Build history of the part. All positions in model axes, mm. A direction names the side the tool comes from. Coordinates: 2 decimals unless noted, no trailing zeros. Loops run counter-clockwise (first coordinate to the right, second up) from the corner with the lowest first, then second, coordinate; pieces in that order, holes last.
(1) Slice it at C-C (y = 89.5). Give the cut face in (x, z), and give its area (3 significant figures).
(2) Slice it at B-B (x = 14.5). Give the number of separate pieces and of enclosed holes in the cut face, and give its area (3 significant figures).
(3) Two-plate mould, pull along Z, no slides. Class faces 1 (the face through (8.87, 60.54, 91.88)), 2 (the face through (9, 50, 249)), 3 (the face through (18, 38, 246)), 4 (the face through (8.87, 60.54, 408.12)): pulls with the +Z half, pulls with the -Z half, needs draft (parallel to the pull), parting line crosses it, or undercut.
(4) Flat gauge pins, fed straight in: P1, Ø5.5, axis at x = 6, y = 82.5, coming from the +Z side; P2, Ø8, axis at x = 13.5, z = 299, coming from the +Y side; P3, Ø1, axis at x = 10, y = 63, coming from the -Z side. Where does each tip first touch, or does it go through?
(5) Tool access for faces 5 (the face through (9, 75, 194.5)), 6 (the face through (9, 100, 313)): list every direction of +Z, -Z, +X, -X, +Y, -Y with a clear straight run to the whole face (end or side of a thin tool).
(6) Wall check: L1, parallel to Y at x = 7.5, z = 314.5; L2, parallel to Z at x = 4.5, y = 29; L3, parallel to Z at x = 6.75, y = 69. Give the ranges that are in metal, low to high.
(7) Slice it at A-A (y = 71). Give the cut face in (x, z), and give its area (3 significant figures).
(8) Slice it at D-D (z = 212.5). Give the cut face in (x, y), and give its area (3 significant figures).
from build123d import *

# Parameters (mm, degrees)
SKETCH1_W                                  = 18
SKETCH1_H                                  = 100
BASE_DEPTH                                 = 500
SKETCH2_W                                  = 111
SKETCH2_H                                  = 50
LAP_JOINT_CUTOUT_DEPTH                     = 511.219560582
LAP_JOINT_BOLT_HOLE_PATTERN_D              = 3.175
CHAMFER_FRONT_SIZE                         = 176.5
CHAMFER_FRONT_SIZE2                        = 82.303301664
CHAMFER_REAR_SIZE                          = 176.5
CHAMFER_REAR_SIZE2                         = 82.303301664
BREAK_CHAMFER_OUTER_CORNERS_R              = 20
CROSS_TIE_BOLT_HOLE_PATTERN_D              = 3.175
FILLET1_R                                  = 10
FLOATING_BEARING_BLOCK_BOLT_HOLE_PATTERN_D = 3.175


with BuildPart() as part:
    # Sketch1 → base (new body)
    with BuildSketch(Plane.XY):
        with Locations((9, 50)):
            Rectangle(SKETCH1_W, SKETCH1_H)
    extrude(amount=BASE_DEPTH)

    # Sketch2 → lap joint cutout (cut, through all)
    with BuildSketch(Plane.ZY):
        with Locations((250, 75)):
            Rectangle(SKETCH2_W, SKETCH2_H)
    extrude(amount=-LAP_JOINT_CUTOUT_DEPTH, mode=Mode.SUBTRACT)

    # lap joint bolt hole pattern (through all)
    with Locations(Plane(origin=(18, 0, 0), x_dir=(0, 0, -1), z_dir=(1, 0, 0))):
        with Locations((-296.5, 40), (-203.5, 10), (-296.5, 10), (-203.5, 40)):
            Hole(LAP_JOINT_BOLT_HOLE_PATTERN_D / 2)

    # chamfer front
    chamfer_front_edges = [part.edges().sort_by_distance(p)[0] for p in [
        (9, 100, 0),
    ]]
    chamfer_front_side = [part.faces().sort_by_distance(p)[0] for p in [
        (9, 100, 97.25),
    ]]
    chamfer(chamfer_front_edges, length=CHAMFER_FRONT_SIZE, length2=CHAMFER_FRONT_SIZE2, reference=chamfer_front_side[0])

    # chamfer rear
    chamfer_rear_edges = [part.edges().sort_by_distance(p)[0] for p in [
        (9, 100, 500),
    ]]
    chamfer_rear_side = [part.faces().sort_by_distance(p)[0] for p in [
        (9, 100, 402.75),
    ]]
    chamfer(chamfer_rear_edges, length=CHAMFER_REAR_SIZE, length2=CHAMFER_REAR_SIZE2, reference=chamfer_rear_side[0])

    # break chamfer outer corners
    break_chamfer_outer_corners_edges = [part.edges().sort_by_distance(p)[0] for p in [
        (9, 17.696698336, 0),
        (9, 17.696698336, 500),
    ]]
    fillet(break_chamfer_outer_corners_edges, radius=BREAK_CHAMFER_OUTER_CORNERS_R)

    # cross tie bolt hole pattern (through all)
    with Locations(Plane(origin=(18, 0, 0), x_dir=(0, 0, -1), z_dir=(1, 0, 0))):
        with Locations((-314.5, 40), (-314.5, 10)):
            cross_tie_bolt_hole_pattern = Hole(CROSS_TIE_BOLT_HOLE_PATTERN_D / 2)

    # mirror cross tie bolt hole pattern: cross tie bolt hole pattern across plane
    add(cross_tie_bolt_hole_pattern.mirror(Plane(origin=(0, 0, 250), x_dir=(1, 0, 0), z_dir=(0, 0, -1))), mode=Mode.SUBTRACT)

    # Fillet1
    fillet1_edges = [part.edges().sort_by_distance(p)[0] for p in [
        (9, 100, 176.5),
        (9, 100, 323.5),
    ]]
    fillet(fillet1_edges, radius=FILLET1_R)

    # floating bearing block bolt hole pattern (through all)
    with Locations(Plane(origin=(18, 0, 0), x_dir=(0, 0, -1), z_dir=(1, 0, 0))):
        with Locations((-268, 30), (-232, 30)):
            Hole(FLOATING_BEARING_BLOCK_BOLT_HOLE_PATTERN_D / 2)


solid = part.part
Response values:
1. outline: (0, 153.98) - (18, 153.98) - (18, 194.5) - (0, 194.5) - close; (0, 305.5) - (18, 305.5) - (18, 346.02) - (0, 346.02) - close
1. area: 1,460 mm2
2. separate pieces: 1
2. enclosed holes: 10
2. area: 29,800 mm2
3. face 1: pulls with the -Z half
3. face 2: undercut
3. face 3: needs draft
3. face 4: pulls with the +Z half
4. P1: stops at z = 366.93
4. P2: stops at y = 50
4. P3: stops at z = 96.08
5. face 5: +X, -X, +Y
5. face 6: +Z, -Z, +X, -X, +Y
6. L1: y = 0 to 8.41, 11.59 to 38.41, 41.59 to 100
6. L2: z = 24.24 to 230.77, 233.23 to 266.77, 269.23 to 475.76
6. L3: z = 110.02 to 194.5, 305.5 to 389.98
7. outline: (0, 114.31) - (18, 114.31) - (18, 194.5) - (0, 194.5) - close; (0, 305.5) - (18, 305.5) - (18, 385.69) - (0, 385.69) - close
7. area: 2,890 mm2
8. outline: (0, 0) - (18, 0) - (18, 50) - (0, 50) - close
8. area: 900 mm2
